Check sheet for the modelled part. Datum: model origin and axes. Units: mm. Round coordinates to 2 decimals unless told otherwise and drop trailing zeros. Order: outer loops, then holes, each group sorted by start corner. A loop starts at its lowest first (then second) coordinate and runs counter-clockwise, first axis right, second up. Notation, with made-up numbers: M 1.25,-19 L 27.25,-19 A36 cw 27.25,19 Z; hole C 26.5,25 d6. An arc over 180 degrees is marked long. One line per item, written item: value. Start each with the question number.
(1) Cross-section at B-B, the plane x = 0.5. Enter the section's corners in (y, z).
(2) Depth check by flat-ended pin: pin 1 Ø1.5 at (y, z) = (-18, 1) entering from -X; pin 2 Ø1.5 at (y, z) = (103, 1.5) entering from -X; pin 3 Ø1.5 at (x, z) = (-62.5, 1.5) entering from +Y. Enter the tip coordinate at first touch or a pass-through.
(3) Thickness scan on L1, parallel to Y at x = -21, z = 1.25; L2, parallel to Y at x = 43, z = 0.9; L3, parallel to Y at x = -4, z = 0.75. Record the ranges inside material, lowest first.
(4) Cross-section at C-C, the plane y = -27.5. Enter the section's corners in (x, z).
(5) Cross-section at A-A, the plane z = 1.05. Count the separate pieces of the cut face and the enclosed holes in it, and give its area (3 significant figures).
from build123d import *

# Parameters (mm, degrees)
SKETCH1_W           = 20
SKETCH1_H           = 3
BOSS_EXTRUDE1_DEPTH = 3


with BuildPart() as part:
    # Sketch1 → Boss-Extrude1 (new body)
    with BuildSketch(Plane.XY):
        Polygon((62.274694919, 0), (62.274694919, -11), (59.274694919, -11), (59.274694919, -31), (62.274694919, -31), (62.274694919, -53), (59.274694919, -53), (59.274694919, -73), (62.274694919, -73), (62.274694919, -84), (-63.725305081, -84), (-63.725305081, -73), (-60.725305081, -73), (-60.725305081, -53), (-63.725305081, -53), (-63.725305081, -31), (-60.725305081, -31), (-60.725305081, -11), (-63.725305081, -11), (-63.725305081, 0), (-57.260838987, 6.464466094), (-55.139518643, 4.343145751), (-48.068450831, 11.414213562), (-50.189771175, 13.535533906), (-43.725305081, 20), (-50.189771175, 26.464466094), (-48.068450831, 28.585786438), (-55.139518643, 35.656854249), (-57.260838987, 33.535533906), (-63.725305081, 40), (-63.725305081, 52), (-60.725305081, 52), (-60.725305081, 72), (-63.725305081, 72), (-63.725305081, 84), (-52.885556553, 91.226499019), (-51.221455964, 88.730348136), (-42.90095302, 94.277350098), (-44.565053609, 96.773500981), (-33.725305081, 104), (-10.725305081, 104), (-10.725305081, 101), (9.274694919, 101), (9.274694919, 104), (32.274694919, 104), (43.114443447, 96.773500981), (41.450342859, 94.277350098), (49.770845802, 88.730348136), (51.434946391, 91.226499019), (62.274694919, 84), (62.274694919, 72), (59.274694919, 72), (59.274694919, 52), (62.274694919, 52), (62.274694919, 40), (55.810228825, 33.535533906), (53.688908482, 35.656854249), (46.61784067, 28.585786438), (48.739161013, 26.464466094), (42.274694919, 20), (48.739161013, 13.535533906), (46.61784067, 11.414213562), (53.688908482, 4.343145751), (55.810228825, 6.464466094), align=None)
        with Locations((29.274694919, -80.5)):
            Rectangle(SKETCH1_W, SKETCH1_H, mode=Mode.SUBTRACT)
        with Locations((-30.725305081, -80.5)):
            Rectangle(SKETCH1_W, SKETCH1_H, mode=Mode.SUBTRACT)
        with Locations((29.274694919, 67)):
            Rectangle(SKETCH1_W, SKETCH1_H, mode=Mode.SUBTRACT)
        with Locations((-30.725305081, 67)):
            Rectangle(SKETCH1_W, SKETCH1_H, mode=Mode.SUBTRACT)
    extrude(amount=BOSS_EXTRUDE1_DEPTH)


solid = part.part
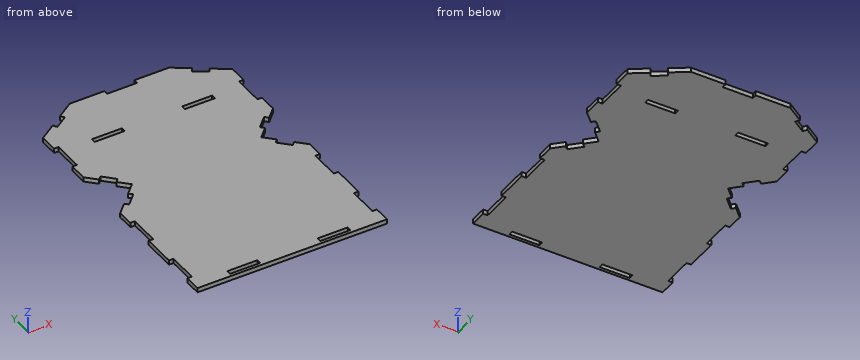
Values found:
1. outline: M -84,0 L 101,0 L 101,3 L -84,3 Z
2. pin 1: x = -60.73
2. pin 2: x = -36.35
2. pin 3: y = 85.32
3. L1: -84 to -82, -79 to 65.5, 68.5 to 104
3. L2: -84 to 19.27, 20.73 to 93.24, 96.6 to 96.85
3. L3: -84 to 101
4. outline: M -60.73,0 L 59.27,0 L 59.27,3 L -60.73,3 Z
5. separate pieces: 1
5. enclosed holes: 4
5. area: 21,400 mm^2
